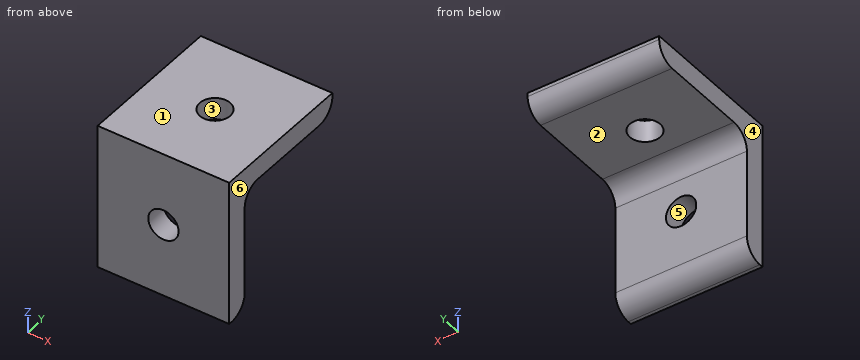
from build123d import *

# Parameters (mm, degrees)
BOSS_EXTRUDE1_DEPTH = 18
SKETCH2_R           = 4.15
CUT_EXTRUDE1_DEPTH  = 7
SKETCH3_R           = 4.15
CUT_EXTRUDE2_DEPTH  = 7
FILLET1_R           = 5


with BuildPart() as part:
    # Sketch1 → Boss-Extrude1 (new body, symmetric)
    with BuildSketch(Plane(origin=(0, 0, 0), x_dir=(0, 0, -1), z_dir=(1, 0, 0))):
        Polygon((0, 40), (0, 0), (40, 0), (40, 6), (6, 6), (6, 40), align=None)
    extrude(amount=BOSS_EXTRUDE1_DEPTH, both=True)

    # Sketch2 → Cut-Extrude1 (cut, through all)
    with BuildSketch(Plane(origin=(0, 6, 0), x_dir=(1, 0, 0), z_dir=(0, 1, 0))):
        with Locations((0, 20)):
            Circle(SKETCH2_R)
    extrude(amount=-CUT_EXTRUDE1_DEPTH, mode=Mode.SUBTRACT)

    # Sketch3 → Cut-Extrude2 (cut, through all)
    with BuildSketch(Plane(origin=(0, 0, -6), x_dir=(-1, 0, 0), z_dir=(0, 0, -1))):
        with Locations((0, 20)):
            Circle(SKETCH3_R)
    extrude(amount=-CUT_EXTRUDE2_DEPTH, mode=Mode.SUBTRACT)

    # Fillet1
    fillet1_edges = [part.edges().sort_by_distance(p)[0] for p in [
        (0, 40, -6),
        (0, 6, -6),
        (0, 6, -40),
    ]]
    fillet(fillet1_edges, radius=FILLET1_R)


solid = part.part
The listing builds one solid part. Answer for the finished solid, in the listing's coordinates (mm). Face numbers are marked on the shaded views. A direction names the side the tool comes from. Coordinates: 2 decimals unless noted, no trailing zeros. Write each loop counter-clockwise with the first axis right and the second up, starting at its lowest first coordinate (ties: lowest second). Pieces come first, ordered by that corner, then holes. Notation, with made-up numbers: (37.25, 73) - (77.25, 73) arc R15 cw to (77.25, 93) - close; hole circle Ø8 at (-38.75, 24). An arc over 180 degrees is marked (long way). Put each result on its own line as item: value.
1. Flat-ended cylindrical pins translate along their axes: pin 1 Ø10 at (x, y) = (-5.5, 32.5) entering from -Z; pin 2 Ø6.5 at (x, y) = (0, 20) entering from +Z; pin 3 Ø7 at (x, z) = (5, -18) entering from +Y; pin 4 Ø3 at (x, y) = (10, 10) entering from -Z. Find the tip coordinate at first contact, or state that the pin passes through.
Answer sheet:
pin 1: stops at z = -6
pin 2: passes through
pin 3: stops at y = 6
pin 4: stops at z = -6.67
2. The part is cut by section A-A on z = -20. Give the vertices of the cut face in (x, y), plus the area to 3 significant figures.
Answer sheet:
outline: (-18, 0) - (-4.15, 0) - (-4.15, 6) - (-18, 6) - close; (4.15, 0) - (18, 0) - (18, 6) - (4.15, 6) - close
area: 166 mm^2
3. A tool of negligible diameter and unlimited length cuts with its end or side. For the marked faces 1 and 2, from which of +Z, -Z, +X, -X, +Y, -Y can it reach the whole face along a straight path? Write none if from no direction.
Answer sheet:
face 1: +Z, +X, -X, +Y, -Y
face 2: -Z, +X, -X, +Y
4. Determine the mould class of the marked faces 3, 4, 5 and 6 for opening direction X: pulls with the +X half, pulls with the -X half, needs draft (parallel to the pull), parting line crosses it, or undercut.
Answer sheet:
face 3: undercut
face 4: pulls with the -X half
face 5: undercut
face 6: pulls with the +X half
5. Find the intervals of material crossed by line 1 along Y through (x, z) = (0, -1.35); line 2 along X through (y, z) = (1.5, -20); line 3 along Y through (x, z) = (9, -20.5), in increasing order. Write a range as from..to.
Answer sheet:
line 1: y = 0..15.85, 24.15..39.99
line 2: x = -18..-4.15, 4.15..18
line 3: y = 0..6
6. The part is cut by section D-D on z = -4. Give the vertices of the cut face in (x, y), plus the area to 3 significant figures.
Answer sheet:
outline: (-18, 0) - (18, 0) - (18, 39) - (-18, 39) - close; hole circle Ø8.3 at (0, 20)
area: 1,350 mm^2
7. The part is cut by section C-C on x = -6. Give the vertices of the cut face in (y, z).
Answer sheet:
outline: (0, -40) - (1, -40) arc R5 ccw to (6, -35) - (6, -11) arc R5 cw to (11, -6) - (35, -6) arc R5 ccw to (40, -1) - (40, 0) - (0, 0) - close
8. The part is cut by section B-B on y = 20. Give the vertices of the cut face in (x, z), plus the area to 3 significant figures.
Answer sheet:
outline: (-18, -6) - (-4.15, -6) - (-4.15, 0) - (-18, 0) - close; (4.15, -6) - (18, -6) - (18, 0) - (4.15, 0) - close
area: 166 mm^2
